Here's how the part is built. I have some questions about the finished solid (model axes, mm). Face numbers are marked on the shaded views. Coordinates: 2 decimals unless noted, no trailing zeros. Order: outer loops, then holes, each group sorted by start corner. A loop starts at its lowest first (then second) coordinate and runs counter-clockwise, first axis right, second up. Notation, with made-up numbers: (22.5, -28.5) - (74.5, -28.5) arc R29 cw to (74.5, -6.5) - close; hole circle Ø8 at (-38, 9.5). An arc over 180 degrees is marked (long way). Answer as CSV lines item,"result". Start each with the question number.
Q1. Suppose I cut it at D-D (x = 83.5). Please give me the cut outline in (y, z), then the cut area to 3 significant figures.
Q2. Suppose I cut it at A-A (z = -53). Please give me the cut outline in (x, y).
Q3. Suppose I cut it at B-B (x = 62.5). Please give me the cut outline in (y, z), then the cut area to 3 significant figures.
Q4. Suppose I cut it at C-C (z = 7). Please give me the cut outline in (x, y), then the cut area to 3 significant figures.
Q5. I need wall thicknesses on line 1 (Y direction, x = 114, z = -59); line 2 (Y direction, x = 76, z = -15); line 3 (X direction, y = 7, z = -46). Which ranges of each line are inside material? Lowest first, please.
Q6. For pin 1 Ø4 at (x, y) = (21.5, 5) entering from -Z; pin 2 Ø2 at (y, z) = (1.5, 4) entering from -X; pin 3 Ø1.2 at (y, z) = (-2, -29.5) entering from +X; pin 4 Ø4 at (x, y) = (50.06, 6.3) entering from +Z, each with a flat end and sliding along its axis, tell me the tip position at first contact or that it passes through.
Q7. Thinking about a two-plate mould opening in X: for the marked faces 1 and 2, which applies, released by +X, released by -X, zero draft, split by the parting line, or undercut?
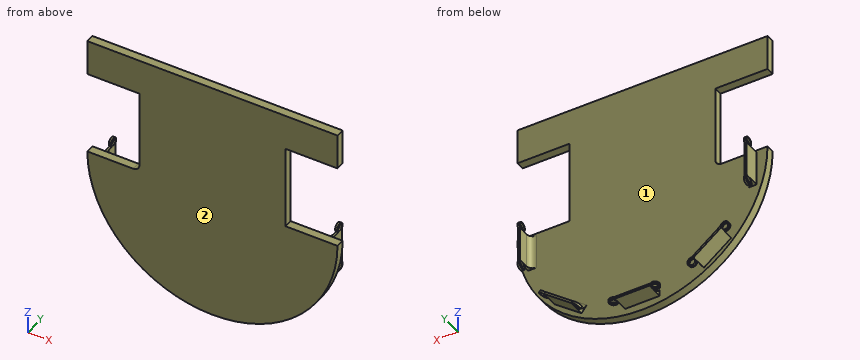
from build123d import *

# Parameters (mm, degrees)
BOSS_EXTRUDE1_DEPTH  = 4
FILLET1_R            = 3
SKETCH3_W            = 1
SKETCH3_H            = 16.52
BOSS_EXTRUDE2_DEPTH  = 8
SKETCH4_R            = 2.1
BOSS_EXTRUDE3_DEPTH  = 1
SKETCH5_R            = 1.6
CUT_EXTRUDE1_DEPTH   = 1
SKETCH6_R            = 2.1
BOSS_EXTRUDE4_DEPTH  = 1
SKETCH7_R            = 1.6
CUT_EXTRUDE2_DEPTH   = 1
FILLET2_R            = 3
SKETCH8_W            = 1
SKETCH8_H            = 16.52
BOSS_EXTRUDE5_DEPTH  = 8
FILLET3_R            = 3
SKETCH9_R            = 2.1
BOSS_EXTRUDE6_DEPTH  = 1
SKETCH10_R           = 2.1
BOSS_EXTRUDE7_DEPTH  = 1
SKETCH11_R           = 1.6
CUT_EXTRUDE3_DEPTH   = 1
SKETCH13_W           = 16.52
SKETCH13_H           = 1
BOSS_EXTRUDE8_DEPTH  = 8
BOSS_EXTRUDE9_DEPTH  = 8
BOSS_EXTRUDE10_DEPTH = 8
SKETCH16_R           = 2.1
BOSS_EXTRUDE11_DEPTH = 1
SKETCH17_R           = 2.1
BOSS_EXTRUDE12_DEPTH = 1
SKETCH18_R           = 1.6
CUT_EXTRUDE4_DEPTH   = 1
SKETCH19_R           = 1.6
CUT_EXTRUDE5_DEPTH   = 1
SKETCH20_R           = 2.1
BOSS_EXTRUDE13_DEPTH = 1
SKETCH21_R           = 2.1
BOSS_EXTRUDE14_DEPTH = 1
SKETCH22_R           = 1.6
CUT_EXTRUDE6_DEPTH   = 1
SKETCH23_R           = 2.1
BOSS_EXTRUDE15_DEPTH = 1
SKETCH24_R           = 2.1
BOSS_EXTRUDE16_DEPTH = 1
SKETCH25_R           = 1.6
CUT_EXTRUDE7_DEPTH   = 1
FILLET4_R            = 3


with BuildPart() as part:
    # Sketch2 → Boss-Extrude1 (new body)
    with BuildSketch(Plane(origin=(0, 0, 0), x_dir=(1, 0, 0), z_dir=(0, 1, 0))):
        with BuildLine():
            Line((0, 0), (0, -17))
            Line((0, -17), (120, -17))
            Line((120, -17), (120, 0))
            Line((120, 0), (95, 0))
            Line((95, 0), (95, 40))
            Line((95, 40), (120, 40))
            ThreePointArc((120, 40), (60, 100), (0, 40))
            Line((0, 40), (25, 40))
            Line((25, 40), (25, 0))
            Line((25, 0), (0, 0))
        make_face()
    extrude(amount=-BOSS_EXTRUDE1_DEPTH)

    # Fillet1
    fillet1_edges = [part.edges().sort_by_distance(p)[0] for p in [
        (25, -2, -40),
    ]]
    fillet(fillet1_edges, radius=FILLET1_R)

    # Sketch3 → Boss-Extrude2 (add)
    with BuildSketch(Plane(origin=(0, 0, 0), x_dir=(1, 0, 0), z_dir=(0, 1, 0))):
        with Locations((5.712890466, 49.353267214)):
            Rectangle(SKETCH3_W, SKETCH3_H)
    extrude(amount=BOSS_EXTRUDE2_DEPTH)

    # Sketch4 → Boss-Extrude3 (add)
    with BuildSketch(Plane.ZY.offset(-5.212890466)):
        with Locations((-59.293267214, 6.3)):
            Circle(SKETCH4_R)
    extrude(amount=-BOSS_EXTRUDE3_DEPTH)

    # Sketch5 → Cut-Extrude1 (cut)
    with BuildSketch(Plane.ZY.offset(-5.212890466)):
        with Locations((-59.293267214, 6.3)):
            Circle(SKETCH5_R)
    extrude(amount=-CUT_EXTRUDE1_DEPTH, mode=Mode.SUBTRACT)

    # Sketch6 → Boss-Extrude4 (add)
    with BuildSketch(Plane.ZY.offset(-5.212890466)):
        with Locations((-39.413267214, 6.3)):
            Circle(SKETCH6_R)
    extrude(amount=-BOSS_EXTRUDE4_DEPTH)

    # Sketch7 → Cut-Extrude2 (cut)
    with BuildSketch(Plane.ZY.offset(-5.212890466)):
        with Locations((-39.413267214, 6.3)):
            Circle(SKETCH7_R)
    extrude(amount=-CUT_EXTRUDE2_DEPTH, mode=Mode.SUBTRACT)

    # Fillet2
    fillet2_edges = [part.edges().sort_by_distance(p)[0] for p in [
        (6.212890466, 0, -49.353267214),
    ]]
    fillet(fillet2_edges, radius=FILLET2_R)

    # Sketch8 → Boss-Extrude5 (add)
    with BuildSketch(Plane(origin=(0, 0, 0), x_dir=(1, 0, 0), z_dir=(0, 1, 0))):
        with Locations((114.29, 49.35)):
            Rectangle(SKETCH8_W, SKETCH8_H)
    extrude(amount=BOSS_EXTRUDE5_DEPTH)

    # Fillet3
    fillet3_edges = [part.edges().sort_by_distance(p)[0] for p in [
        (113.79, 0, -49.35),
    ]]
    fillet(fillet3_edges, radius=FILLET3_R)

    # Sketch9 → Boss-Extrude6 (add)
    with BuildSketch(Plane(origin=(114.79, 0, 0), x_dir=(0, 0, -1), z_dir=(1, 0, 0))):
        with Locations((39.41, 6.3)):
            Circle(SKETCH9_R)
    extrude(amount=-BOSS_EXTRUDE6_DEPTH)

    # Sketch10 → Boss-Extrude7 (add)
    with BuildSketch(Plane(origin=(114.79, 0, 0), x_dir=(0, 0, -1), z_dir=(1, 0, 0))):
        with Locations((59.29, 6.3)):
            Circle(SKETCH10_R)
    extrude(amount=-BOSS_EXTRUDE7_DEPTH)

    # Sketch11 → Cut-Extrude3 (cut)
    with BuildSketch(Plane(origin=(114.79, 0, 0), x_dir=(0, 0, -1), z_dir=(1, 0, 0))):
        with Locations((39.41, 6.3)):
            Circle(SKETCH11_R)
        with Locations((59.29, 6.3)):
            Circle(SKETCH11_R)
    extrude(amount=-CUT_EXTRUDE3_DEPTH, mode=Mode.SUBTRACT)

    # Sketch13 → Boss-Extrude8 (add)
    with BuildSketch(Plane(origin=(0, 0, 0), x_dir=(1, 0, 0), z_dir=(0, 1, 0))):
        with Locations((60, 95.723174162)):
            Rectangle(SKETCH13_W, SKETCH13_H)
    extrude(amount=BOSS_EXTRUDE8_DEPTH)

    # Sketch14 → Boss-Extrude9 (add)
    with BuildSketch(Plane(origin=(0, 0, 0), x_dir=(1, 0, 0), z_dir=(0, 1, 0))):
        Polygon((102.309314854, 79.933135701), (89.191434032, 89.974629751), (88.583595409, 89.180569168), (101.701476231, 79.139075118), align=None)
    extrude(amount=BOSS_EXTRUDE9_DEPTH)

    # Sketch15 → Boss-Extrude10 (add)
    with BuildSketch(Plane(origin=(0, 0, 0), x_dir=(1, 0, 0), z_dir=(0, 1, 0))):
        Polygon((30.495980982, 90.292754217), (17.38126662, 80.247124958), (17.989355558, 79.45325605), (31.104069921, 89.498885309), align=None)
    extrude(amount=BOSS_EXTRUDE10_DEPTH)

    # Sketch16 → Boss-Extrude11 (add)
    with BuildSketch(Plane(origin=(0, 0, -96.223174162), x_dir=(-1, 0, 0), z_dir=(0, 0, -1))):
        with Locations((-69.94, 6.3)):
            Circle(SKETCH16_R)
    extrude(amount=-BOSS_EXTRUDE11_DEPTH)

    # Sketch17 → Boss-Extrude12 (add)
    with BuildSketch(Plane(origin=(0, 0, -96.223174162), x_dir=(-1, 0, 0), z_dir=(0, 0, -1))):
        with Locations((-50.06, 6.3)):
            Circle(SKETCH17_R)
    extrude(amount=-BOSS_EXTRUDE12_DEPTH)

    # Sketch18 → Cut-Extrude4 (cut)
    with BuildSketch(Plane(origin=(0, 0, -96.223174162), x_dir=(-1, 0, 0), z_dir=(0, 0, -1))):
        with Locations((-69.94, 6.3)):
            Circle(SKETCH18_R)
    extrude(amount=-CUT_EXTRUDE4_DEPTH, mode=Mode.SUBTRACT)

    # Sketch19 → Cut-Extrude5 (cut)
    with BuildSketch(Plane(origin=(0, 0, -96.223174162), x_dir=(-1, 0, 0), z_dir=(0, 0, -1))):
        with Locations((-50.06, 6.3)):
            Circle(SKETCH19_R)
    extrude(amount=-CUT_EXTRUDE5_DEPTH, mode=Mode.SUBTRACT)

    # Sketch20 → Boss-Extrude13 (add)
    with BuildSketch(Plane(origin=(76.380579105, 0, -99.781101182), x_dir=(-0.7940605824226628, 0, -0.607838622861843), z_dir=(0.6078386228618429, 0, -0.7940605824226626))):
        with Locations((-34.333347015, 6.3)):
            Circle(SKETCH20_R)
    extrude(amount=-BOSS_EXTRUDE13_DEPTH)

    # Sketch21 → Boss-Extrude14 (add)
    with BuildSketch(Plane(origin=(76.380579105, 0, -99.781101182), x_dir=(-0.7940605824226628, 0, -0.607838622861843), z_dir=(0.6078386228618429, 0, -0.7940605824226626))):
        with Locations((-14.453347015, 6.3)):
            Circle(SKETCH21_R)
    extrude(amount=-BOSS_EXTRUDE14_DEPTH)

    # Sketch22 → Cut-Extrude6 (cut)
    with BuildSketch(Plane(origin=(76.380579105, 0, -99.781101182), x_dir=(-0.7940605824226628, 0, -0.607838622861843), z_dir=(0.6078386228618429, 0, -0.7940605824226626))):
        with Locations((-34.333347015, 6.3)):
            Circle(SKETCH22_R)
        with Locations((-14.453347015, 6.3)):
            Circle(SKETCH22_R)
    extrude(amount=-CUT_EXTRUDE6_DEPTH, mode=Mode.SUBTRACT)

    # Sketch23 → Boss-Extrude15 (add)
    with BuildSketch(Plane(origin=(-32.311621485, 0, -42.183289414), x_dir=(-0.7938689081223455, 0, 0.6080889381633537), z_dir=(-0.6080889381633537, 0, -0.7938689081223455))):
        with Locations((-80.79583616, 6.3)):
            Circle(SKETCH23_R)
    extrude(amount=-BOSS_EXTRUDE15_DEPTH)

    # Sketch24 → Boss-Extrude16 (add)
    with BuildSketch(Plane(origin=(-32.311621485, 0, -42.183289414), x_dir=(-0.7938689081223455, 0, 0.6080889381633537), z_dir=(-0.6080889381633537, 0, -0.7938689081223455))):
        with Locations((-60.91583616, 6.3)):
            Circle(SKETCH24_R)
    extrude(amount=-BOSS_EXTRUDE16_DEPTH)

    # Sketch25 → Cut-Extrude7 (cut)
    with BuildSketch(Plane(origin=(-32.311621485, 0, -42.183289414), x_dir=(-0.7938689081223455, 0, 0.6080889381633537), z_dir=(-0.6080889381633537, 0, -0.7938689081223455))):
        with Locations((-80.79583616, 6.3)):
            Circle(SKETCH25_R)
        with Locations((-60.91583616, 6.255190771)):
            Circle(SKETCH25_R)
    extrude(amount=-CUT_EXTRUDE7_DEPTH, mode=Mode.SUBTRACT)

    # Fillet4
    fillet4_edges = [part.edges().sort_by_distance(p)[0] for p in [
        (60, 0, -95.223174162),
        (95.14253582, 0, -84.159822143),
        (24.54671274, 0, -84.47607068),
    ]]
    fillet(fillet4_edges, radius=FILLET4_R)


solid = part.part
Here are the results:
1,outline,"(-4, -95.21) - (0, -95.21) - (0, 17) - (-4, 17) - close"
1,area,"449 mm²"
2,outline,"(1.43, -4) - (118.57, -4) - (118.57, 0) - (114.79, 0) - (114.79, 8) - (113.79, 8) - (113.79, 3) arc R3 cw to (110.79, 0) - (9.21, 0) arc R3 cw to (6.21, 3) - (6.21, 8) - (5.21, 8) - (5.21, 0) - (1.43, 0) - close"
3,outline,"(-4, -99.95) - (0, -99.95) - (0, -96.22) - (8, -96.22) - (8, -95.22) - (3, -95.22) arc R3 cw to (0, -92.22) - (0, 17) - (-4, 17) - close"
3,area,"478 mm²"
4,outline,"(0, -4) - (120, -4) - (120, 0) - (0, 0) - close"
4,area,"480 mm²"
5,line 1,"y = -4 to 0, 4.22 to 4.73, 7.87 to 8.38"
5,line 2,"y = -4 to 0"
5,line 3,"x = 5.21 to 6.21, 113.79 to 114.79"
6,pin 1,"stops at z = -84.93"
6,pin 2,"passes through"
6,pin 3,"stops at x = 95"
6,pin 4,"stops at z = -95.22"
7,face 1,"undercut"
7,face 2,"zero draft"
